For this review, take the finished solid that the model builds, in its own axes (mm). A direction names the side the tool comes from. Give positions to 0.01 mm unless a question says otherwise; leave off trailing zeros. Loops run counter-clockwise (first coordinate to the right, second up) from the corner with the lowest first, then second, coordinate; pieces in that order, holes last. Notation, with made-up numbers: (-27, 2) - (13, 2) arc R35 cw to (13, 38) - close; hole circle Ø8 at (12.25, 14.5). An arc over 180 degrees is marked (long way). Use CSV: the item, a comma, the result in double quotes. Start each with the question number.
1. For faces 1 (the flat face through (-21, -3.81, 2)), 2 (the flat face through (21, 3.81, 2)), 3 (the flat face through (-3.81, -21, 2)), 4 (the flat face through (-3.81, 21, 2)), list the 3-axis set-ups (+Z, -Z, +X, -X, +Y, -Y) from which the entire face can be reached by the end or side of a thin tool; tool diameter is ignored.
2. Take a section at B-B on z = 2. Give the boundary of the cut face in (x, y) (1 decimal), plus the area to 3 significant figures.
3. Mouldability with a two-part tool opening along X and no side actions: class faces 5 (the flat face through (21, -3.81, 2)), 6 (the cylindrical face through (-5.175, -31.325, 1.565)), 7 (the cylindrical face through (6.39, -0.08, 1.57)), 8 (the cylindrical face through (-3.78, -2.9, 1.57)) as pulls with the +X half, pulls with the -X half, needs draft (parallel to the pull), parting line crosses it, or undercut.
4. Take a section at A-A on x = 0. Give the boundary of the cut face in (y, z) (1 decimal).
5. Wall thickness on line 1 (Y direction, x = 28, z = 1.45); line 2 (Y direction, x = 0, z = 2.25); line 3 (X direction, y = 24.5, z = 2.85): over which ranges is each line inside the solid? List them lowest first.
6. For pin 1 (1 mm diameter, centred on x = -19.5, z = 1.5, fed in from -Y); pin 2 (7.5 mm diameter, centred on x = 0, y = 0, fed in from -Z); pin 3 (1.5 mm diameter, centred on y = 5.5, z = 2.5, fed in from +X); pin 4 (1 mm diameter, centred on x = 16, z = 2, fed in from +Y), all flat-tipped, find the tip position at first contact; note any pin that passes through.
```python
from build123d import *

# Parameters (mm, degrees)
F0_R     = 4.7625
F1_DEPTH = 3.175


with BuildPart() as f1:
    # F0 (on Top) → F1 (new body)
    with BuildSketch(Plane.XY):
        with BuildLine():
            ThreePointArc((-6.49331, 31.078922), (-12.572359, 12.572359), (-31.078922, 6.49331))
            ThreePointArc((-31.078922, 6.49331), (-31.328488, 5.156386), (-31.520571, 3.81))
            Line((-31.520571, 3.81), (-10.200497, 3.81))
            ThreePointArc((-10.200497, 3.81), (-6.390497, 0), (-10.200497, -3.81))
            Line((-10.200497, -3.81), (-31.520571, -3.81))
            ThreePointArc((-31.520571, -3.81), (-31.328488, -5.156386), (-31.078922, -6.49331))
            ThreePointArc((-31.078922, -6.49331), (-12.572359, -12.572359), (-6.49331, -31.078922))
            ThreePointArc((-6.49331, -31.078922), (-5.156386, -31.328488), (-3.81, -31.520571))
            Line((-3.81, -31.520571), (-3.81, -10.200497))
            ThreePointArc((-3.81, -10.200497), (0, -6.390497), (3.81, -10.200497))
            Line((3.81, -10.200497), (3.81, -31.520571))
            ThreePointArc((3.81, -31.520571), (5.156386, -31.328488), (6.49331, -31.078922))
            ThreePointArc((6.49331, -31.078922), (12.572359, -12.572359), (31.078922, -6.49331))
            ThreePointArc((31.078922, -6.49331), (31.328488, -5.156386), (31.520571, -3.81))
            Line((31.520571, -3.81), (10.200497, -3.81))
            ThreePointArc((10.200497, -3.81), (6.390497, 0), (10.200497, 3.81))
            Line((10.200497, 3.81), (31.520571, 3.81))
            ThreePointArc((31.520571, 3.81), (31.328488, 5.156386), (31.078922, 6.49331))
            ThreePointArc((31.078922, 6.49331), (12.572359, 12.572359), (6.49331, 31.078922))
            ThreePointArc((6.49331, 31.078922), (5.156386, 31.328488), (3.81, 31.520571))
            Line((3.81, 31.520571), (3.81, 10.200497))
            ThreePointArc((3.81, 10.200497), (0, 6.390497), (-3.81, 10.200497))
            Line((-3.81, 10.200497), (-3.81, 31.520571))
            ThreePointArc((-3.81, 31.520571), (-5.156386, 31.328488), (-6.49331, 31.078922))
        make_face()
        Circle(F0_R, mode=Mode.SUBTRACT)
    extrude(amount=F1_DEPTH)


solid = f1.part
```
Check result:
1,face 1,"+Z, -Z, -X"
1,face 2,"+Z, -Z, +X"
1,face 3,"+Z, -Z, -Y"
1,face 4,"+Z, -Z, +Y"
2,outline,"(-31.5, -3.8) arc R31.8 ccw to (-31.1, -6.5) arc R21.6 cw to (-6.5, -31.1) arc R31.8 ccw to (-3.8, -31.5) - (-3.8, -10.2) arc R3.8 cw to (3.8, -10.2) - (3.8, -31.5) arc R31.8 ccw to (6.5, -31.1) arc R21.6 cw to (31.1, -6.5) arc R31.8 ccw to (31.5, -3.8) - (10.2, -3.8) arc R3.8 cw to (10.2, 3.8) - (31.5, 3.8) arc R31.8 ccw to (31.1, 6.5) arc R21.6 cw to (6.5, 31.1) arc R31.8 ccw to (3.8, 31.5) - (3.8, 10.2) arc R3.8 cw to (-3.8, 10.2) - (-3.8, 31.5) arc R31.8 ccw to (-6.5, 31.1) arc R21.6 cw to (-31.1, 6.5) arc R31.8 ccw to (-31.5, 3.8) - (-10.2, 3.8) arc R3.8 cw to (-10.2, -3.8) - close; hole circle Ø9.5 at (0, 0)"
2,area,"1,010 mm²"
3,face 5,"needs draft"
3,face 6,"pulls with the -X half"
3,face 7,"pulls with the +X half"
3,face 8,"undercut"
4,outline,"(-6.4, 0) - (-4.8, 0) - (-4.8, 3.2) - (-6.4, 3.2) - close; (4.8, 0) - (6.4, 0) - (6.4, 3.2) - (4.8, 3.2) - close"
5,line 1,"y = -6.25 to -3.81, 3.81 to 6.25"
5,line 2,"y = -6.39 to -4.76, 4.76 to 6.39"
5,line 3,"x = -6.51 to -3.81, 3.81 to 6.51"
6,pin 1,"stops at y = -8.14"
6,pin 2,"passes through"
6,pin 3,"stops at x = 31.39"
6,pin 4,"stops at y = 10.12"
